```python
from build123d import *

# Parameters (mm, degrees)
SKETCH1_W           = 60
SKETCH1_H           = 50
BOSS_EXTRUDE1_DEPTH = 40
SHELL1_T            = 2.2
SKETCH2_W           = 52
SKETCH2_H           = 40
CUT_EXTRUDE1_DEPTH  = 10
SKETCH3_W           = 10
SKETCH3_H           = 10
CUT_EXTRUDE2_DEPTH  = 5
BOSS_EXTRUDE2_DEPTH = 5
CHAMFER3_SIZE       = 5
CHAMFER4_SIZE       = 4
FILLET1_R           = 4


with BuildPart() as part:
    # Sketch1 → Boss-Extrude1 (new body)
    with BuildSketch(Plane(origin=(0, 0, 0), x_dir=(1, 0, 0), z_dir=(0, 1, 0))):
        Rectangle(SKETCH1_W, SKETCH1_H)
    extrude(amount=BOSS_EXTRUDE1_DEPTH)

    # Shell1 (no face opened: a closed hollow body)
    add(offset(amount=-SHELL1_T, mode=Mode.PRIVATE), mode=Mode.SUBTRACT)

    # Sketch2 → Cut-Extrude1 (cut)
    with BuildSketch(Plane(origin=(0, 40, 0), x_dir=(1, 0, 0), z_dir=(0, 1, 0))):
        Rectangle(SKETCH2_W, SKETCH2_H)
    extrude(amount=-CUT_EXTRUDE1_DEPTH, mode=Mode.SUBTRACT)

    # Sketch3 → Cut-Extrude2 (cut)
    with BuildSketch(Plane(origin=(-30, 0, 0), x_dir=(0, 0, -1), z_dir=(1, 0, 0))):
        with Locations((0, 33)):
            Rectangle(SKETCH3_W, SKETCH3_H)
    extrude(amount=CUT_EXTRUDE2_DEPTH, mode=Mode.SUBTRACT)

    # Sketch4 → Boss-Extrude2 (add)
    with BuildSketch(Plane(origin=(-30, 0, 0), x_dir=(0, 0, -1), z_dir=(1, 0, 0))):
        Polygon((-5, 38), (-7, 38), (-7, 26), (7, 26), (7, 38), (5, 38), (5, 28), (-5, 28), align=None)
    extrude(amount=-BOSS_EXTRUDE2_DEPTH)

    # Chamfer3
    chamfer3_edges = [part.edges().sort_by_distance(p)[0] for p in [
        (-30, 26, 0),
    ]]
    chamfer(chamfer3_edges, length=CHAMFER3_SIZE - 0.0001)  # a hair under: the kernel refuses the full size

    # Chamfer4
    chamfer4_edges = [part.edges().sort_by_distance(p)[0] for p in [
        (-31.4, 28, 5),
        (-31.4, 28, -5),
    ]]
    chamfer(chamfer4_edges, length=CHAMFER4_SIZE)

    # Fillet1
    fillet1_edges = [part.edges().sort_by_distance(p)[0] for p in [
        (0, 0, 25),
        (-30, 0, 0),
        (0, 0, -25),
        (30, 0, 0),
    ]]
    fillet(fillet1_edges, radius=FILLET1_R)


solid = part.part
```
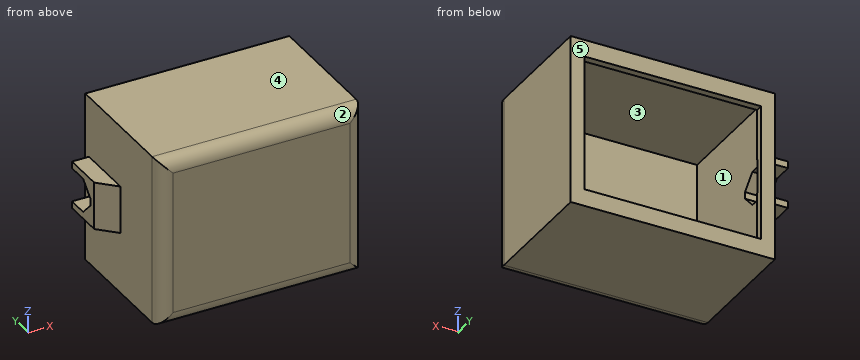
Can you work these out from the model? Positions are in its coordinate system, mm. Face numbers are marked on the shaded views. A direction names the side the tool comes from. Coordinates: 2 decimals unless noted, no trailing zeros. Loops run counter-clockwise (first coordinate to the right, second up) from the corner with the lowest first, then second, coordinate; pieces in that order, holes last.
Item 1: Suppose I cut it at D-D (x = 4). Please give me the cut outline in (y, z), then the cut area to 3 significant figures.
Answers below:
outline: (0, -21) arc R4 ccw to (4, -25) - (40, -25) - (40, -20) - (37.8, -20) - (37.8, -22.8) - (2.2, -22.8) - (2.2, 22.8) - (37.8, 22.8) - (37.8, 20) - (40, 20) - (40, 25) - (4, 25) arc R4 ccw to (0, 21) - close
area: 282 mm2
Item 2: Please list where these lines run through material, in increasing order: L1, parallel to Z at x = 21, y = 19.5; L2, parallel to X at y = 38.5, z = -15.5; L3, parallel to X at y = 12.5, z = -4.
Answers below:
L1: z = -25 to -22.8, 22.8 to 25
L2: x = -30 to -26, 26 to 30
L3: x = -30 to -27.8, 27.8 to 30
Item 3: Suppose I cut it at A-A (y = 29.5). Please give me the cut outline in (x, z).
Answers below:
outline: (-35, -7) - (-30, -7) - (-30, -25) - (30, -25) - (30, 25) - (-30, 25) - (-30, 7) - (-35, 7) - (-35, 2.5) - (-27.8, 2.5) - (-27.8, 22.8) - (27.8, 22.8) - (27.8, -22.8) - (-27.8, -22.8) - (-27.8, -2.5) - (-35, -2.5) - close
Item 4: Which directions (+Z, -Z, +X, -X, +Y, -Y) give clear straight access to the entire face, cutting with the end or side of a thin tool? Please do the marked faces 1 and 2.
Answers below:
face 1: none
face 2: +Z, +X, -X, -Y
Item 5: Suppose I cut it at C-C (z = -17.5). Please give me the cut outline in (x, y), then the cut area to 3 significant figures.
Answers below:
outline: (-30, 4) arc R4 ccw to (-26, 0) - (26, 0) arc R4 ccw to (30, 4) - (30, 40) - (26, 40) - (26, 37.8) - (27.8, 37.8) - (27.8, 2.2) - (-27.8, 2.2) - (-27.8, 37.8) - (-26, 37.8) - (-26, 40) - (-30, 40) - close
area: 299 mm2
Item 6: If we mould it in two halves opening along Y, with no side actions, what happens to the marked faces 3, 4 and 5? For each: released by +Y, released by -Y, zero draft, split by the parting line, or undercut.
Answers below:
face 3: undercut
face 4: zero draft
face 5: released by +Y
Item 7: Suppose I cut it at B-B (y = 17). Please give me the cut outline in (x, z), then the cut area to 3 significant figures.
Answers below:
outline: (-30, -25) - (30, -25) - (30, 25) - (-30, 25) - close; hole (-27.8, -22.8) - (27.8, -22.8) - (27.8, 22.8) - (-27.8, 22.8) - close
area: 465 mm2
Item 8: I'm going to push flat-ended pins straight in: pin 1 (1 mm diameter, centred on x = -31.5, z = -6, fed in from +Y); pin 2 (1 mm diameter, centred on y = 33.5, z = 17, fed in from -X); pin 3 (10.5 mm diameter, centred on y = 19, z = -9.5, fed in from -X). Where does each tip first touch, or does it pass through?
Answers below:
pin 1: stops at y = 38
pin 2: stops at x = -30
pin 3: stops at x = -32.62
